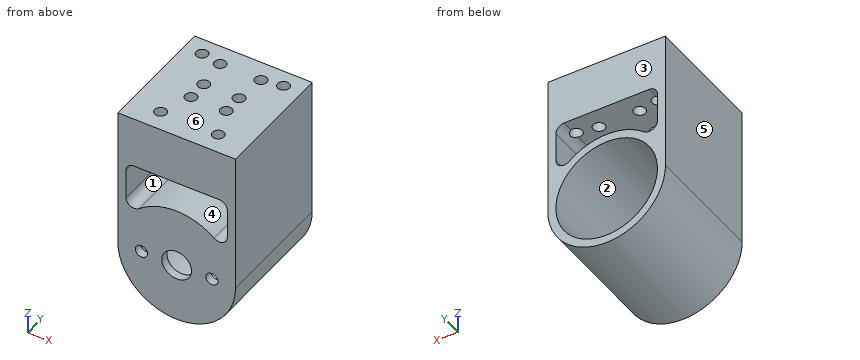
from build123d import *

# Parameters (mm, degrees)
CROQUIS1_R              = 14.45
SALIENTE_EXTRUIR1_DEPTH = 30
CROQUIS3_W              = 28.9
CROQUIS3_H              = 18.45
SALIENTE_EXTRUIR2_DEPTH = 30
CROQUIS4_R              = 12.475
CORTAR_EXTRUIR2_DEPTH   = 28
CROQUIS6_R              = 1.5
CORTAR_EXTRUIR4_DEPTH   = 28
CROQUIS7_R              = 1.45
CORTAR_EXTRUIR5_DEPTH   = 3
CROQUIS8_R              = 3.65
CORTAR_EXTRUIR6_DEPTH   = 2
SALIENTE_EXTRUIR4_START = 16.1
CROQUIS9_W              = 28.9
CROQUIS9_H              = 30
CROQUIS9_R              = 1.45
SALIENTE_EXTRUIR4_DEPTH = 16.1
CORTAR_EXTRUIR7_DEPTH   = 48.984424556


with BuildPart() as part:
    # Croquis1 → Saliente-Extruir1 (new body)
    with BuildSketch(Plane(origin=(0, 0, 0), x_dir=(1, 0, 0), z_dir=(0, 1, 0))):
        with Locations(Location((0, 0, 0), (0, 0, 270))):
            Circle(CROQUIS1_R)
    extrude(amount=SALIENTE_EXTRUIR1_DEPTH)

    # Croquis3 → Saliente-Extruir2 (add)
    with BuildSketch(Plane(origin=(0, 0, 0), x_dir=(1, 0, 0), z_dir=(0, 1, 0))):
        with Locations((0, -9.225)):
            Rectangle(CROQUIS3_W, CROQUIS3_H)
    extrude(amount=SALIENTE_EXTRUIR2_DEPTH)

    # Croquis4 → Cortar-Extruir2 (cut)
    with BuildSketch(Plane(origin=(0, 30, 0), x_dir=(1, 0, 0), z_dir=(0, 1, 0))):
        with Locations(Location((0, 0, 0), (0, 0, 270))):
            Circle(CROQUIS4_R)
    extrude(amount=-CORTAR_EXTRUIR2_DEPTH, mode=Mode.SUBTRACT)

    # Croquis6 → Cortar-Extruir4 (cut)
    with BuildSketch(Plane(origin=(0, 2, 0), x_dir=(1, 0, 0), z_dir=(0, 1, 0))):
        with Locations(Location((8.65, 0, 0), (0, 0, 270))):
            Circle(CROQUIS6_R)
        with Locations(Location((-8.65, 0, 0), (0, 0, 270))):
            Circle(CROQUIS6_R)
    extrude(amount=-CORTAR_EXTRUIR4_DEPTH, mode=Mode.SUBTRACT)

    # Croquis7 → Cortar-Extruir5 (cut)
    with BuildSketch(Plane.XY.offset(18.45)):
        with Locations((-5, 25)):
            Circle(CROQUIS7_R)
        with Locations((5, 25)):
            Circle(CROQUIS7_R)
        with Locations((-7.0711, 5)):
            Circle(CROQUIS7_R)
        with Locations(Location((7.0711, 5, 0), (0, 0, 180))):
            Circle(CROQUIS7_R)
        with Locations((-4.330127019, 17.5)):
            Circle(CROQUIS7_R)
        with Locations(Location((4.330127019, 12.5, 0), (0, 0, 180))):
            Circle(CROQUIS7_R)
        with Locations((-10, 25.88)):
            Circle(CROQUIS7_R)
        with Locations(Location((10, 25.88, 0), (0, 0, 180))):
            Circle(CROQUIS7_R)
        with Locations((-4.330127019, 12.5)):
            Circle(CROQUIS7_R)
        with Locations(Location((4.330127019, 17.5, 0), (0, 0, 180))):
            Circle(CROQUIS7_R)
    extrude(amount=-CORTAR_EXTRUIR5_DEPTH, mode=Mode.SUBTRACT)

    # Croquis8 → Cortar-Extruir6 (cut)
    with BuildSketch(Plane.XZ):
        with Locations(Location((0, 0, 0), (0, 0, 270))):
            Circle(CROQUIS8_R)
    extrude(amount=-CORTAR_EXTRUIR6_DEPTH, mode=Mode.SUBTRACT)

    # Croquis9 → Saliente-Extruir4 (add)
    with BuildSketch(Plane.XY.offset(18.45).offset(SALIENTE_EXTRUIR4_START)):
        with Locations((0, 15)):
            Rectangle(CROQUIS9_W, CROQUIS9_H)
        with Locations((-4.330127019, 12.5)):
            Circle(CROQUIS9_R, mode=Mode.SUBTRACT)
        with Locations((4.330127019, 17.5)):
            Circle(CROQUIS9_R, mode=Mode.SUBTRACT)
        with Locations((-5, 25)):
            Circle(CROQUIS9_R, mode=Mode.SUBTRACT)
        with Locations((5, 25)):
            Circle(CROQUIS9_R, mode=Mode.SUBTRACT)
        with Locations((-7.0711, 5)):
            Circle(CROQUIS9_R, mode=Mode.SUBTRACT)
        with Locations((7.0711, 5)):
            Circle(CROQUIS9_R, mode=Mode.SUBTRACT)
        with Locations((-4.330127019, 17.5)):
            Circle(CROQUIS9_R, mode=Mode.SUBTRACT)
        with Locations((4.330127019, 12.5)):
            Circle(CROQUIS9_R, mode=Mode.SUBTRACT)
        with Locations((-10, 25.88)):
            Circle(CROQUIS9_R, mode=Mode.SUBTRACT)
        with Locations((10, 25.88)):
            Circle(CROQUIS9_R, mode=Mode.SUBTRACT)
    extrude(amount=-SALIENTE_EXTRUIR4_DEPTH)

    # Croquis10 → Cortar-Extruir7 (cut, through all)
    with BuildSketch(Plane(origin=(0, 30, 0), x_dir=(1, 0, 0), z_dir=(0, 1, 0))):
        with BuildLine():
            Line((-10.45, -22), (10.45, -22))
            ThreePointArc((10.45, -22), (11.864213562, -21.414213562), (12.45, -20))
            Line((12.45, -20), (12.45, -12.736684223))
            ThreePointArc((12.45, -12.736684223), (11.305225835, -10.928760339), (9.181411229, -11.190501009))
            ThreePointArc((9.181411229, -11.190501009), (0, -14.475), (-9.181411229, -11.190501009))
            ThreePointArc((-9.181411229, -11.190501009), (-11.305225835, -10.928760339), (-12.45, -12.736684223))
            Line((-12.45, -12.736684223), (-12.45, -20))
            ThreePointArc((-12.45, -20), (-11.864213562, -21.414213562), (-10.45, -22))
        make_face()
    extrude(amount=-CORTAR_EXTRUIR7_DEPTH, mode=Mode.SUBTRACT)


solid = part.part
Check sheet for the modelled part. Datum: model origin and axes. Units: mm. Face numbers are marked on the shaded views. A direction names the side the tool comes from. Round coordinates to 2 decimals unless told otherwise and drop trailing zeros. Order: outer loops, then holes, each group sorted by start corner. A loop starts at its lowest first (then second) coordinate and runs counter-clockwise, first axis right, second up. Notation, with made-up numbers: M 58.25,1.5 L 77.25,1.5 A12 ccw 77.25,6.5 Z; hole C -31.75,-18 d6. An arc over 180 degrees is marked long. One line per item, written item: value. Start each with the question number.
1. Release check for a two-part mould opening along Z. For the marked faces 4, 5 and 6 record: released by +Z, released by -Z, zero draft, split by the parting line, or undercut.
2. Access from +Z, -Z, +X, -X, +Y, -Y to the whole of each face (thin tool, end or side, straight path). Record for the marked faces 1, 2 and 3.
3. Section check C-C on x = -4.5. Enter the section's corners in (y, z).
4. Scan lines: line 1 along Z through (x, y) = (1, 8.5); line 2 along Y through (x, z) = (5.5, 28); line 3 along X through (y, z) = (4, 29). Record each from-to range of solid material in increasing order.
5. Section check B-B on z = 16. Enter the section's corners in (x, y).
6. Section check A-A on y = 17.5. Give the number of separate pieces and of enclosed holes in the cut face, and give its area (3 significant figures).
7. Gauge pin test, flat ends, axial feed: P1, Ø4, axis at x = 4.33, y = 12.5, coming from the -Z side; P2, Ø3.5, axis at x = 8.65, z = 0, coming from the +Y side; P3, Ø4, axis at x = -10, y = 25.88, coming from the -Z side; P4, Ø4.5, axis at x = 0, z = 0, coming from the -Y side (3 decimals). Record the tip position at first contact, or that the pin passes through.
Results found:
1. face 4: undercut
1. face 5: zero draft
1. face 6: released by +Z
2. face 1: +Y, -Y
2. face 2: +Y
2. face 3: +Z, -Z, +X, -X, +Y
3. outline: M 0,-13.73 L 30,-13.73 L 30,-11.64 L 2,-11.64 L 2,11.64 L 30,11.64 L 30,13.76 L 0,13.76 Z; M 0,22 L 11.06,22 L 11.06,34.55 L 0,34.55 Z; M 13.94,22 L 16.06,22 L 16.06,34.55 L 13.94,34.55 Z; M 18.94,22 L 23.64,22 L 23.64,34.55 L 18.94,34.55 Z; M 26.36,22 L 30,22 L 30,34.55 L 26.36,34.55 Z
4. line 1: -14.42 to -12.43, 12.43 to 14.44, 22 to 34.55
4. line 2: 0 to 11.64, 13.36 to 16.64, 18.36 to 23.64, 26.36 to 30
4. line 3: -14.45 to -8.12, -6.02 to 6.02, 8.12 to 14.45
5. outline: M -14.45,0 L -12.45,0 L -12.45,30 L -14.45,30 Z; M 12.45,0 L 14.45,0 L 14.45,30 L 12.45,30 Z
6. separate pieces: 2
6. enclosed holes: 1
6. area: 538 mm^2
7. P1: z = -14.26
7. P2: y = 2
7. P3: z = -12.03
7. P4: through
